from build123d import *

# Parameters (mm, degrees)
IZIM2_R                     = 7.1
IZIM2_R_2                   = 2
IZIM2_R_3                   = 2.1
Y_KSEKLIK_EKSTR_ZYON1_DEPTH = 5.5
IZIM3_R                     = 20.5
KES_EKSTR_ZYON1_DEPTH       = 1.5


with BuildPart() as part:
    # Çizim2 → Yükseklik-Ekstrüzyon1 (new body)
    with BuildSketch(Plane(origin=(0, 0, 0), x_dir=(1, 0, 0), z_dir=(0, 1, 0))):
        with BuildLine():
            Line((-20.15, -24.15), (20.15, -24.15))
            ThreePointArc((20.15, -24.15), (22.978427125, -22.978427125), (24.15, -20.15))
            Line((24.15, -20.15), (24.15, 20.15))
            ThreePointArc((24.15, 20.15), (22.978427125, 22.978427125), (20.15, 24.15))
            Line((20.15, 24.15), (-20.15, 24.15))
            ThreePointArc((-20.15, 24.15), (-22.978427125, 22.978427125), (-24.15, 20.15))
            Line((-24.15, 20.15), (-24.15, -20.15))
            ThreePointArc((-24.15, -20.15), (-22.978427125, -22.978427125), (-20.15, -24.15))
        make_face()
        Circle(IZIM2_R, mode=Mode.SUBTRACT)
        with Locations((-18, 18)):
            Circle(IZIM2_R_2, mode=Mode.SUBTRACT)
        with Locations((18, 18)):
            Circle(IZIM2_R_2, mode=Mode.SUBTRACT)
        with Locations((-18, -18)):
            Circle(IZIM2_R_2, mode=Mode.SUBTRACT)
        with Locations((18, -18)):
            Circle(IZIM2_R_2, mode=Mode.SUBTRACT)
        with Locations((-15.5, 0)):
            Circle(IZIM2_R_3, mode=Mode.SUBTRACT)
        with Locations((15.5, 0)):
            Circle(IZIM2_R_3, mode=Mode.SUBTRACT)
    extrude(amount=Y_KSEKLIK_EKSTR_ZYON1_DEPTH)

    # Çizim3 → Kes-Ekstrüzyon1 (cut)
    with BuildSketch(Plane(origin=(0, 5.5, 0), x_dir=(1, 0, 0), z_dir=(0, 1, 0))):
        Circle(IZIM3_R)
    extrude(amount=-KES_EKSTR_ZYON1_DEPTH, mode=Mode.SUBTRACT)


solid = part.part
The listing builds one solid part. Answer for the finished solid, in the listing's coordinates (mm). A direction names the side the tool comes from. Coordinates: 2 decimals unless noted, no trailing zeros. Order: outer loops, then holes, each group sorted by start corner. A loop starts at its lowest first (then second) coordinate and runs counter-clockwise, first axis right, second up. Notation, with made-up numbers: (22.5, 73.5) -> (72.5, 73.5) arc R27 ccw to (72.5, 112.5) -> close; hole circle Ø8 at (62, 74.5). An arc over 180 degrees is marked (long way). Answer in a Markdown table with one row per item. Add a question column.
Item 1: Find section B-B (y = 2.65). Write down the section's boundary in (x, z), then the cut area to 3 significant figures.
Item 2: Find section D-D (z = 18). Write down the section's boundary in (x, y).
Item 3: Each of these flat-tipped pins is pushed along its axis until it touches: P1, Ø4, axis at x = -15.5, z = -1, coming from the +Y side; P2, Ø5, axis at x = -18, z = -18, coming from the -Y side; P3, Ø2.5, axis at x = 15.5, z = 0, coming from the -Y side. Where does it stop, or does it pass through?
Item 4: Find the intervals of material crossed by L1, parallel to X at y = 1.3, z = 0; L2, parallel to Z at x = 18, y = 2.8, in increasing order. Write a range as from..to.
Item 5: Find section A-A (z = 0). Write down the section's boundary in (x, y), then the cut area to 3 significant figures.
Item 6: Find section C-C (x = 0). Write down the section's boundary in (y, z).
Item 7: Determine the mould class of faces 1 (the face through (18, 3, 16)), 2 (the face through (0, 3, 24.15)), 3 (the face through (-23.009, 2.712, 22.947)) for opening direction X: +X half, -X half, draft (parallel to the pull), parting line (faces both ways), or undercut.
Item 8: Which of the six approach directions +Z, -Z, +X, -X, +Y, -Y give full straight-line access (tool end or side, diameter ignored) to faces 4 (the face through (9, 4, 0)), 5 (the face through (-24.15, 3, 0))?
Result set:
| question | item | result |
|---|---|---|
| 1 | outline | (-24.15, -20.15) arc R4 ccw to (-20.15, -24.15) -> (20.15, -24.15) arc R4 ccw to (24.15, -20.15) -> (24.15, 20.15) arc R4 ccw to (20.15, 24.15) -> (-20.15, 24.15) arc R4 ccw to (-24.15, 20.15) -> close; hole circle Ø4 at (-18, -18); hole circle Ø4 at (-18, 18); hole circle Ø4.2 at (-15.5, 0); hole circle Ø14.2 at (0, 0); hole circle Ø4.2 at (15.5, 0); hole circle Ø4 at (18, -18); hole circle Ø4 at (18, 18) |
| 1 | area | 2,080 mm² |
| 2 | outline | (-24.15, 0) -> (-20, 0) -> (-20, 5.5) -> (-24.15, 5.5) -> close; (-16, 0) -> (16, 0) -> (16, 5.5) -> (9.81, 5.5) -> (9.81, 4) -> (-9.81, 4) -> (-9.81, 5.5) -> (-16, 5.5) -> close; (20, 0) -> (24.15, 0) -> (24.15, 5.5) -> (20, 5.5) -> close |
| 3 | P1 | stops at y = 4 |
| 3 | P2 | stops at y = 0 |
| 3 | P3 | passes through |
| 4 | L1 | x = -24.15..-17.6, -13.4..-7.1, 7.1..13.4, 17.6..24.15 |
| 4 | L2 | z = -24.15..-20, -16..16, 20..24.15 |
| 5 | outline | (-24.15, 0) -> (-17.6, 0) -> (-17.6, 4) -> (-20.5, 4) -> (-20.5, 5.5) -> (-24.15, 5.5) -> close; (-13.4, 0) -> (-7.1, 0) -> (-7.1, 4) -> (-13.4, 4) -> close; (7.1, 0) -> (13.4, 0) -> (13.4, 4) -> (7.1, 4) -> close; (17.6, 0) -> (24.15, 0) -> (24.15, 5.5) -> (20.5, 5.5) -> (20.5, 4) -> (17.6, 4) -> close |
| 5 | area | 114 mm² |
| 6 | outline | (0, -24.15) -> (5.5, -24.15) -> (5.5, -20.5) -> (4, -20.5) -> (4, -7.1) -> (0, -7.1) -> close; (0, 7.1) -> (4, 7.1) -> (4, 20.5) -> (5.5, 20.5) -> (5.5, 24.15) -> (0, 24.15) -> close |
| 7 | face 1 | undercut |
| 7 | face 2 | draft |
| 7 | face 3 | -X half |
| 8 | face 4 | +Y |
| 8 | face 5 | +Z, -Z, -X, +Y, -Y |
